from build123d import *

# Parameters (mm, degrees)
SKETCH1_R           = 22.5
BOSS_EXTRUDE1_DEPTH = 15
SKETCH3_R           = 22.5
CUT_EXTRUDE1_DEPTH  = 43
SKETCH4_R           = 37
SKETCH4_R_2         = 32
BOSS_EXTRUDE2_DEPTH = 15


with BuildPart() as part:
    # Sketch1 → Boss-Extrude1 (new body)
    with BuildSketch(Plane.XY):
        Circle(SKETCH1_R)
    extrude(amount=BOSS_EXTRUDE1_DEPTH)

    # Sketch2 → Revolve1 (revolve)
    with BuildSketch(Plane(origin=(0, 0, 0), x_dir=(0, 0, -1), z_dir=(1, 0, 0))):
        Polygon((-15, 49), (-15, 22.5), (-10, 22.5), (-10, 48.592881079), (0, 109.592881079), (0, 110), (-5, 110), align=None)
    revolve(axis=Axis((0, 0, 15), (0, 0, -1)))

    # Sketch3 → Cut-Extrude1 (cut)
    with BuildSketch(Plane.XY.offset(15)):
        Circle(SKETCH3_R)
    extrude(amount=-CUT_EXTRUDE1_DEPTH, mode=Mode.SUBTRACT)

    # Sketch4 → Boss-Extrude2 (add)
    with BuildSketch(Plane(origin=(0, 0, 10), x_dir=(-1, 0, 0), z_dir=(0, 0, -1))):
        Circle(SKETCH4_R)
        Circle(SKETCH4_R_2, mode=Mode.SUBTRACT)
    extrude(amount=BOSS_EXTRUDE2_DEPTH)


solid = part.part
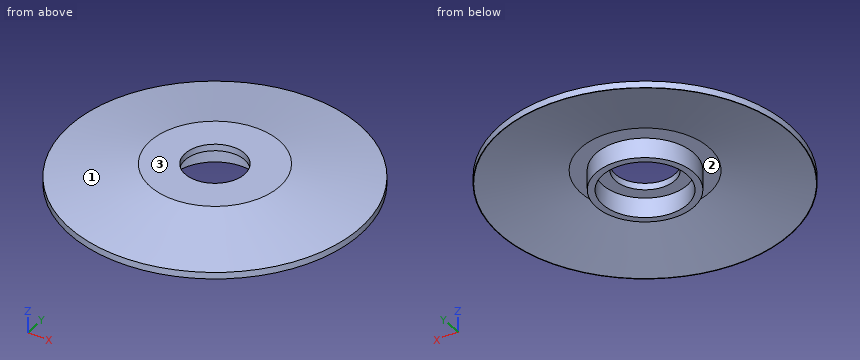
Geometry check sheet. Reference: the model listing, model coordinates, mm. Face numbers are marked on the shaded views. Give positions to 0.01 mm unless a question says otherwise; leave off trailing zeros. Loops run counter-clockwise (first coordinate to the right, second up) from the corner with the lowest first, then second, coordinate; pieces in that order, holes last. Notation, with made-up numbers: M 63.5,-7.75 L 114.5,-7.75 A22 ccw 114.5,12.25 Z; hole C -22.75,85.25 d7. An arc over 180 degrees is marked long. Answer as a JSON object with one key per item and string values. Group by question number.
Item 1: Mould release check, pull along X, two halves, no side actions. Record for the marked faces 1, 2 and 3: pulls with the +X half, pulls with the -X half, needs draft (parallel to the pull), parting line crosses it, or undercut.
Item 2: Gauge pin test, flat ends, axial feed: pin 1 (1.5 mm diameter, centred on x = 34, z = 2, fed in from +Y); pin 2 (12 mm diameter, centred on x = 20, y = 50, fed in from -Z); pin 3 (8 mm diameter, centred on y = -81.5, z = 5.5, fed in from -X); pin 4 (1.5 mm diameter, centred on x = -76.5, z = 12.5, fed in from +Y). Record the tip position at first contact, or that the pin passes through.
Item 3: Sectioned sample at C-C on z = -2.5. Record the boundary of the cut face in (x, y), plus the area to 3 significant figures.
Item 4: Sectioned sample at A-A on x = 0. Record the boundary of the cut face in (y, z), plus the area to 3 significant figures.
Item 5: Material ranges on L1, parallel to Y at x = 0, z = -0.25; L2, parallel to Z at x = 46, y = 11; L3, parallel to Y at x = -6.5, z = -1.75, recorded low to high.
Findings below:
{
 "1": {"face 1": "parting line crosses it", "face 2": "undercut", "face 3": "needs draft"},
 "2": {"pin 1": "y = 104.85", "pin 2": "z = 8.15", "pin 3": "x = -78.03", "pin 4": "through"},
 "3": {"outline": "C 0,0 d74; hole C 0,0 d64", "area": "1,080 mm2"},
 "4": {"outline": "M -110,0 L -109.59,0 L -48.59,10 L -37,10 L -37,-5 L -32,-5 L -32,10 L -22.5,10 L -22.5,15 L -49,15 L -110,5 Z; M 22.5,10 L 32,10 L 32,-5 L 37,-5 L 37,10 L 48.59,10 L 109.59,0 L 110,0 L 110,5 L 49,15 L 22.5,15 Z", "area": "1,030 mm2"},
 "5": {"L1": "-37 to -32, 32 to 37", "L2": "10 to 15", "L3": "-36.42 to -31.33, 31.33 to 36.42"}
}
